The figure shows three views and two pictorial views of one solid part (mm, origin at its lowest corner). Answer the questions. Coordinates: 2 decimals unless noted, no trailing zeros. Write each loop counter-clockwise with the first axis right and the second up, starting at its lowest first coordinate (ties: lowest second). Pieces come first, ordered by that corner, then holes. Notation, with made-up numbers: M 88,45 L 105,45 A20 ccw 105,72 Z; hole C 40,38 d2. An arc over 180 degrees is marked long. Write item = value, one per line.
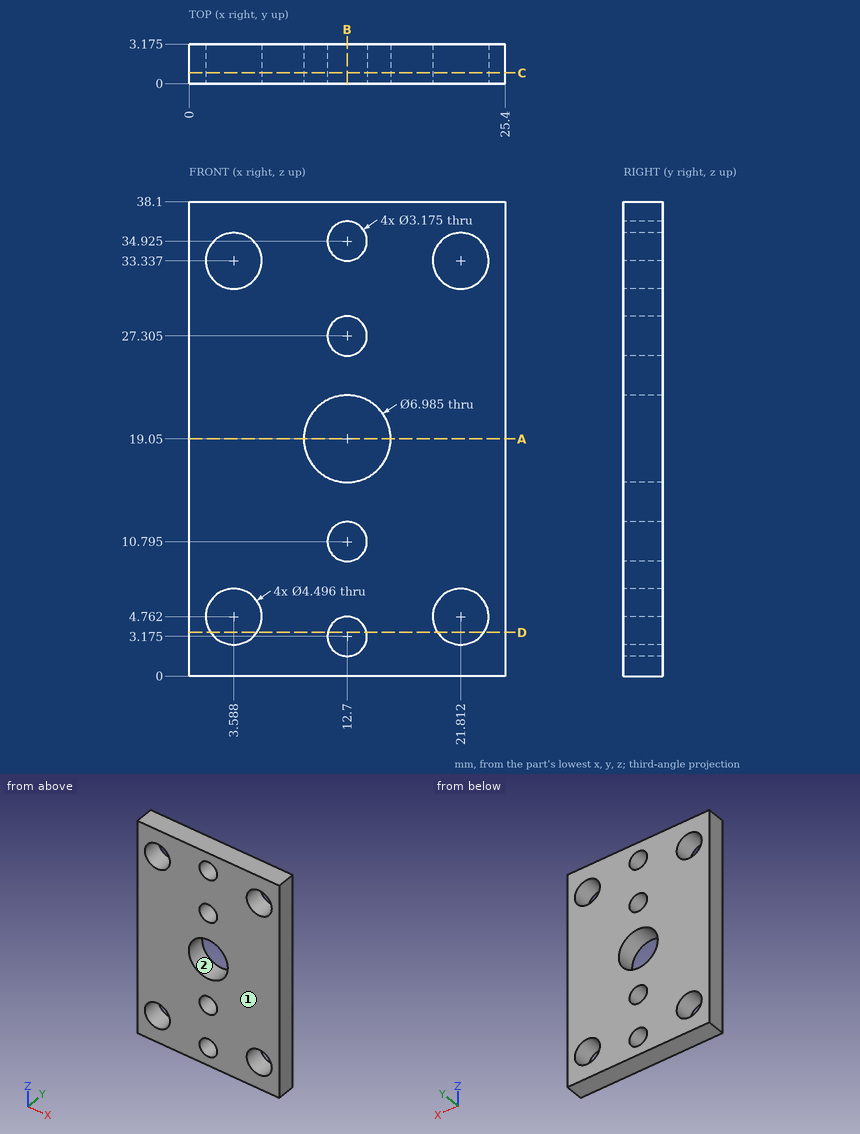
Item 1: A flat-ended cylindrical pin translates along its axis: pin 1 (2.5 mm diameter, centred on x = 3.59, z = 4.76, fed in from -Y). Find the tip coordinate at first contact, or state that the pin passes through.
Worked answers:
pin_1 = through
Item 2: Find section A-A (z = 19.05). Determine the outline of the cut face in (x, y) (1 decimal).
Worked answers:
outline = M 0,0 L 9.2,0 L 9.2,3.2 L 0,3.2 Z; M 16.2,0 L 25.4,0 L 25.4,3.2 L 16.2,3.2 Z
Item 3: Find section C-C (y = 0.85). State how many separate pieces and enclosed holes the cut face has, and give its area (3 significant figures).
Worked answers:
separate_pieces = 1
enclosed_holes = 9
area = 834 mm²
Item 4: Find section B-B (x = 12.7). Determine the outline of the cut face in (y, z) (1 decimal).
Worked answers:
outline = M 0,0 L 3.2,0 L 3.2,1.6 L 0,1.6 Z; M 0,4.8 L 3.2,4.8 L 3.2,9.2 L 0,9.2 Z; M 0,12.4 L 3.2,12.4 L 3.2,15.6 L 0,15.6 Z; M 0,22.5 L 3.2,22.5 L 3.2,25.7 L 0,25.7 Z; M 0,28.9 L 3.2,28.9 L 3.2,33.3 L 0,33.3 Z; M 0,36.5 L 3.2,36.5 L 3.2,38.1 L 0,38.1 Z
Item 5: Find section D-D (z = 3.5). Determine the outline of the cut face in (x, y) (1 decimal).
Worked answers:
outline = M 0,0 L 1.7,0 L 1.7,3.2 L 0,3.2 Z; M 5.4,0 L 11.1,0 L 11.1,3.2 L 5.4,3.2 Z; M 14.3,0 L 20,0 L 20,3.2 L 14.3,3.2 Z; M 23.7,0 L 25.4,0 L 25.4,3.2 L 23.7,3.2 Z
Item 6: Consider line 1 along Z through (x, y) = (12.7, 2); line 2 along Z through (x, y) = (12.25, 0.75) (1 decimal); line 3 along Z through (x, y) = (21.5, 2.8). Determine where each line is inside the solid, lowest interval first. Write a range as from..to.
Worked answers:
line_1 = 0..1.59, 4.76..9.21, 12.38..15.56, 22.54..25.72, 28.89..33.34, 36.51..38.1
line_2 = 0..1.7, 4.7..9.3, 12.3..15.6, 22.5..25.8, 28.8..33.4, 36.4..38.1
line_3 = 0..2.54, 6.99..31.11, 35.56..38.1
Item 7: For a pull along X with two mould halves and no side action, classify the marked faces 1 and 2 as released by +X, released by -X, zero draft, split by the parting line, or undercut.
Worked answers:
face_1 = zero draft
face_2 = undercut
